The model under review builds one solid part; all positions refer to its coordinate system, in mm. A direction names the side the tool comes from. Round coordinates to 2 decimals unless told otherwise and drop trailing zeros. Write each loop counter-clockwise with the first axis right and the second up, starting at its lowest first coordinate (ties: lowest second). Pieces come first, ordered by that corner, then holes. Notation, with made-up numbers: (56, 77) - (89, 77) arc R30 cw to (89, 102) - close; hole circle Ø6 at (31.5, -9). An arc over 180 degrees is marked (long way). Return JSON: item names as keys, results as strings.
from build123d import *

# Parameters (mm, degrees)
SKETCH1_W                                         = 25.4
SKETCH1_H                                         = 6
SKETCH2_R                                         = 15
BOSS_EXTRUDE1_DEPTH                               = 56.2
CUT_EXTRUDE1_DEPTH                                = 63.2
SKETCH4_W                                         = 7.0104
SKETCH4_H                                         = 65.418639441
F_2_CLEARANCE_HOLE1_D                             = 2.5
F_2_CLEARANCE_HOLE1_DEPTH                         = 12
SKETCH7_W                                         = 1.25
SKETCH7_H                                         = 16.341500105
CSK_FOR_8_FLAT_HEAD_MACHINE_SCREW_100_D           = 4.5
CSK_FOR_8_FLAT_HEAD_MACHINE_SCREW_100_DEPTH       = 62.2
CSK_FOR_8_FLAT_HEAD_MACHINE_SCREW_100_CSINK_D     = 9.4
CSK_FOR_8_FLAT_HEAD_MACHINE_SCREW_100_CSINK_ANGLE = 90
SKETCH11_R                                        = 10.3124
CUT_EXTRUDE2_DEPTH                                = 38.1


with BuildPart() as part:
    # Sketch1 → Revolve1 (revolve)
    with BuildSketch(Plane.XZ):
        with Locations((12.7, 58.54)):
            Rectangle(SKETCH1_W, SKETCH1_H)
    revolve(axis=Axis((0, 0, 61.54), (0, 0, -1)))

    # Sketch2 → Boss-Extrude1 (add)
    with BuildSketch(Plane(origin=(0, 0, 55.54), x_dir=(-1, 0, 0), z_dir=(0, 0, -1))):
        Circle(SKETCH2_R)
    extrude(amount=BOSS_EXTRUDE1_DEPTH)

    # Sketch3 → Cut-Extrude1 (cut, through all)
    with BuildSketch(Plane(origin=(0, 0, -0.66), x_dir=(-1, 0, 0), z_dir=(0, 0, -1))):
        with BuildLine():
            Line((2.5, 9.058499895), (-2.5, 9.058499895))
            Line((-2.5, 9.058499895), (-2.5, 6.538348415))
            ThreePointArc((-2.5, 6.538348415), (0, 7), (2.5, 6.538348415))
            Line((2.5, 6.538348415), (2.5, 9.058499895))
        make_face()
    extrude(amount=-CUT_EXTRUDE1_DEPTH, mode=Mode.SUBTRACT)

    # Sketch4 → Cut-Revolve1 (revolve, cut)
    with BuildSketch(Plane.XZ):
        with Locations((3.5052, 28.83068028)):
            Rectangle(SKETCH4_W, SKETCH4_H)
    revolve(axis=Axis((0, 0, 61.54), (0, 0, -1)), mode=Mode.SUBTRACT)

    # #2 Clearance Hole1
    with Locations(Plane(origin=(0, 0, -0.66), x_dir=(-1, 0, 0), z_dir=(0, 0, -1))):
        with Locations((-11.5, 0), (-5.75, -9.959292144), (5.75, -9.959292144), (11.5, 0), (5.75, 9.959292144), (-5.75, 9.959292144)):
            Hole(F_2_CLEARANCE_HOLE1_D / 2, depth=F_2_CLEARANCE_HOLE1_DEPTH)

    # Sketch7 → #2 Clearance Hole2 (revolve, cut)
    with BuildSketch(Plane(origin=(0, 9.058499895, 20.422), x_dir=(0, 0, -1), z_dir=(1, 0, 0))):
        with Locations((0.625, 8.170750053)):
            Rectangle(SKETCH7_W, SKETCH7_H)
    revolve(axis=Axis((0, 2.708499895, 20.422), (0, 1, 0)), mode=Mode.SUBTRACT)

    # CSK for #8 Flat Head Machine Screw (100)1
    with Locations(Plane.XY.offset(61.54)):
        with Locations((0, 20.4), (14.424978336, 14.424978336), (20.4, 0), (14.424978336, -14.424978336), (0, -20.4), (-14.424978336, -14.424978336), (-20.4, 0), (-14.424978336, 14.424978336)):
            CounterSinkHole(CSK_FOR_8_FLAT_HEAD_MACHINE_SCREW_100_D / 2, CSK_FOR_8_FLAT_HEAD_MACHINE_SCREW_100_CSINK_D / 2, depth=CSK_FOR_8_FLAT_HEAD_MACHINE_SCREW_100_DEPTH, counter_sink_angle=CSK_FOR_8_FLAT_HEAD_MACHINE_SCREW_100_CSINK_ANGLE)

    # Sketch11 → Cut-Extrude2 (cut)
    with BuildSketch(Plane.XY.offset(61.54)):
        Circle(SKETCH11_R)
    extrude(amount=-CUT_EXTRUDE2_DEPTH, mode=Mode.SUBTRACT)


solid = part.part
(1) Add section A-A (y = -20.4). Write out the cut boundary in (x, z).
Filled in:
{"outline": "(-15.13, 55.54) - (-2.25, 55.54) - (-2.25, 59.09) - (-4.7, 61.54) - (-15.13, 61.54) - close; (2.25, 55.54) - (15.13, 55.54) - (15.13, 61.54) - (4.7, 61.54) - (2.25, 59.09) - close"}
(2) Add section B-B (x = 5.75). Write out the cut boundary in (y, z).
Filled in:
{"outline": "(-24.74, 55.54) - (-13.85, 55.54) - (-13.85, -0.66) - (-11.21, -0.66) - (-11.21, 11.34) - (-8.71, 11.34) - (-8.71, -0.66) - (-4.01, -0.66) - (-4.01, 23.44) - (-8.56, 23.44) - (-8.56, 61.54) - (-24.74, 61.54) - close; (4.01, -0.66) - (8.71, -0.66) - (8.71, 11.34) - (11.21, 11.34) - (11.21, -0.66) - (13.85, -0.66) - (13.85, 55.54) - (24.74, 55.54) - (24.74, 61.54) - (8.56, 61.54) - (8.56, 23.44) - (4.01, 23.44) - close"}
(3) Clearance check with flat-ended pins moving along their axes: pin 1 Ø5 at (x, z) = (2.5, 15.5) entering from +Y; pin 2 Ø1.2 at (x, y) = (-6.5, -9.5) entering from -Z; pin 3 Ø1.2 at (x, y) = (6, -10) entering from -Z; pin 4 Ø8 at (x, z) = (-7.5, 27) entering from -Y. State where each tip first meets the part, or that it passes through.
Filled in:
{"pin 1": "stops at y = 15", "pin 2": "stops at z = -0.66", "pin 3": "stops at z = 11.34", "pin 4": "stops at y = -14.59"}
(4) Wall thickness on line 1 (Y direction, x = 0, z = 57); line 2 (Y direction, x = -5, z = 4); line 3 (Z direction, x = 0, y = 11): over which ranges is each line inside the solid? List them lowest first.
Filled in:
{"line 1": "y = -25.4 to -22.65, -18.15 to -10.31, 10.31 to 18.15, 22.65 to 25.4", "line 2": "y = -14.14 to -10.96, -8.96 to -4.91, 4.91 to 8.96, 10.96 to 14.14", "line 3": "z = -0.66 to 19.17, 21.67 to 61.54"}
(5) Mouldability with a two-part tool opening along Y and no side actions: class faces 5 (the flat face through (0, 11, 61.54)), 6 (the conical face through (12.165, 15.137, 59.209)) as released by +Y, released by -Y, zero draft, split by the parting line, or undercut.
Filled in:
{"face 5": "zero draft", "face 6": "undercut"}
(6) Add section D-D (z = 31.5). Write out the cut boundary in (x, y).
Filled in:
{"outline": "circle Ø30 at (0, 0); hole circle Ø20.62 at (0, 0)"}
(7) Add section C-C (z = 20.5). Write out the cut boundary in (x, y), plus the area to 3 significant figures.
Filled in:
{"outline": "(-2.5, 6.55) - (-2.5, 9.06) - (-1.25, 9.06) - (-1.25, 14.95) arc R15 ccw (long way) to (1.25, 14.95) - (1.25, 9.06) - (2.5, 9.06) - (2.5, 6.55) arc R7.01 cw (long way) to start", "area": "527 mm2"}
(8) For faces 1 (the flat face through (-2.5, 8, 11)), 2 (the cylindrical face through (5.54, 8.7, 42.76)), 3 (the flat face through (-3.1, -6.5, -0.66)), 4 (the flat face through (6, 10, 11.34)), list the 3-axis set-ups (+Z, -Z, +X, -X, +Y, -Y) from which the entire face can be reached by the end or side of a thin tool; tool diameter is ignored.
Filled in:
{"face 1": "+Z, -Z", "face 2": "+Z", "face 3": "-Z, +X, -X, +Y, -Y", "face 4": "-Z"}
